```python
from build123d import *

# Parameters (mm, degrees)
SKETCH1_W                = 34
SKETCH1_H                = 28.5
BOSS_EXTRUDE1_DEPTH      = 22.7
SKETCH3_R                = 12.6
CUT_EXTRUDE1_DEPTH       = 21
SKETCH5_R                = 1.625
SKETCH5_R_2              = 3.75
CUT_EXTRUDE2_DEPTH       = 31.546071761
BOSS_EXTRUDE2_DEPTH      = 4.93
BOSS_EXTRUDE2_DEPTH_BACK = 3.72
SKETCH7_W                = 8.75
SKETCH7_H                = 12.5
SKETCH8_R                = 1.75
CUT_EXTRUDE3_DEPTH       = 42.018037496
SKETCH9_R                = 3.25
CUT_EXTRUDE4_DEPTH       = 3.175
SKETCH14_R               = 1.75
CUT_EXTRUDE8_DEPTH       = 50


with BuildPart() as part:
    # Sketch1 → Boss-Extrude1 (new body)
    with BuildSketch(Plane.XY):
        Rectangle(SKETCH1_W, SKETCH1_H)
    extrude(amount=BOSS_EXTRUDE1_DEPTH)

    # Sketch3 → Cut-Extrude1 (cut)
    with BuildSketch(Plane.XY.offset(22.7)):
        Circle(SKETCH3_R)
    extrude(amount=-CUT_EXTRUDE1_DEPTH, mode=Mode.SUBTRACT)

    # Sketch5 → Cut-Extrude2 (cut, through all)
    with BuildSketch(Plane.XY.offset(1.7)):
        with Locations((6.01040764, 6.01040764)):
            Circle(SKETCH5_R)
        with Locations((-6.01040764, 6.01040764)):
            Circle(SKETCH5_R)
        with Locations((6.01040764, -6.01040764)):
            Circle(SKETCH5_R)
        with Locations((-6.01040764, -6.01040764)):
            Circle(SKETCH5_R)
        Circle(SKETCH5_R_2)
    extrude(amount=-CUT_EXTRUDE2_DEPTH, mode=Mode.SUBTRACT)

    # Sketch7 → Boss-Extrude2 (add, two sides: drawn at the far end of the back side and taken through both)
    with BuildSketch(Plane.XY.offset(22.7).offset(-BOSS_EXTRUDE2_DEPTH_BACK)):
        with Locations((-21.375, -8)):
            Rectangle(SKETCH7_W, SKETCH7_H)
        with Locations((21.375, -8)):
            Rectangle(SKETCH7_W, SKETCH7_H)
    extrude(amount=BOSS_EXTRUDE2_DEPTH + BOSS_EXTRUDE2_DEPTH_BACK)

    # Sketch8 → Cut-Extrude3 (cut, through all)
    with BuildSketch(Plane(origin=(0, -1.75, 0), x_dir=(1, 0, 0), z_dir=(0, 1, 0))):
        with Locations(Location((21.375, -23.305, 0), (0, 0, 180))):
            Circle(SKETCH8_R)
        with Locations(Location((-21.375, -23.305, 0), (0, 0, 180))):
            Circle(SKETCH8_R)
    extrude(amount=-CUT_EXTRUDE3_DEPTH, mode=Mode.SUBTRACT)

    # Sketch9 → Cut-Extrude4 (cut)
    with BuildSketch(Plane.XZ.offset(14.25)):
        with Locations((-21.375, 23.305)):
            Circle(SKETCH9_R)
        with Locations((21.375, 23.305)):
            Circle(SKETCH9_R)
    extrude(amount=-CUT_EXTRUDE4_DEPTH, mode=Mode.SUBTRACT)

    # Cut-Extrude5 cone 1 section (through the dimple's axis) → Cut-Extrude5 (revolve, cut)
    with BuildSketch(Plane(origin=(-6.01040764, 6.01040764, 0), x_dir=(0, 1, 0), z_dir=(1, 0, 0))):
        Polygon((0, 0), (2.8, 0), (0, 2.8), align=None)
    revolve(axis=Axis((-6.01040764, 6.01040764, 0), (0, 0, 1)), mode=Mode.SUBTRACT)

    # Cut-Extrude5 cone 2 section (through the dimple's axis) → Cut-Extrude5 cone 2 (revolve, cut)
    with BuildSketch(Plane(origin=(-6.01040764, -6.01040764, 0), x_dir=(0, 1, 0), z_dir=(1, 0, 0))):
        Polygon((0, 0), (2.8, 0), (0, 2.8), align=None)
    revolve(axis=Axis((-6.01040764, -6.01040764, 0), (0, 0, 1)), mode=Mode.SUBTRACT)

    # Cut-Extrude5 cone 3 section (through the dimple's axis) → Cut-Extrude5 cone 3 (revolve, cut)
    with BuildSketch(Plane(origin=(6.01040764, -6.01040764, 0), x_dir=(0, 1, 0), z_dir=(1, 0, 0))):
        Polygon((0, 0), (2.8, 0), (0, 2.8), align=None)
    revolve(axis=Axis((6.01040764, -6.01040764, 0), (0, 0, 1)), mode=Mode.SUBTRACT)

    # Cut-Extrude5 cone 4 section (through the dimple's axis) → Cut-Extrude5 cone 4 (revolve, cut)
    with BuildSketch(Plane(origin=(6.01040764, 6.01040764, 0), x_dir=(0, 1, 0), z_dir=(1, 0, 0))):
        Polygon((0, 0), (2.8, 0), (0, 2.8), align=None)
    revolve(axis=Axis((6.01040764, 6.01040764, 0), (0, 0, 1)), mode=Mode.SUBTRACT)

    # Sketch14 → Cut-Extrude8 (cut)
    with BuildSketch(Plane(origin=(132.323959999, 1.25, 25.756345109), x_dir=(1, 0, 0), z_dir=(0, 1, 0))):
        with Locations((-110.733959999, 2.481345109)):
            Circle(SKETCH14_R)
        with Locations((-153.913959999, 2.481345109)):
            Circle(SKETCH14_R)
    extrude(amount=-CUT_EXTRUDE8_DEPTH, mode=Mode.SUBTRACT)


solid = part.part
```
Part model, mm, in its own coordinate system. A direction names the side the tool comes from. Round coordinates to 2 decimals unless told otherwise and drop trailing zeros. Write each loop counter-clockwise with the first axis right and the second up, starting at its lowest first coordinate (ties: lowest second). Pieces come first, ordered by that corner, then holes.
Item 1: Cut at C-C, the plane z = 26. Give the cut face in (x, y) (3 decimals), plus the area to 3 significant figures.
Results:
outline: (-25.75, -14.25) - (-23.191, -14.25) - (-23.191, -11.075) - (-19.559, -11.075) - (-19.559, -14.25) - (-17, -14.25) - (-17, -1.75) - (-25.75, -1.75) - close; (17, -14.25) - (19.559, -14.25) - (19.559, -11.075) - (23.191, -11.075) - (23.191, -14.25) - (25.75, -14.25) - (25.75, -1.75) - (17, -1.75) - close
area: 196 mm2
Item 2: Cut at A-A, the plane x = 0. Give the cut face in (y, z), plus the area to 3 significant figures.
Results:
outline: (-14.25, 0) - (-3.75, 0) - (-3.75, 1.7) - (-12.6, 1.7) - (-12.6, 22.7) - (-14.25, 22.7) - close; (3.75, 0) - (14.25, 0) - (14.25, 22.7) - (12.6, 22.7) - (12.6, 1.7) - (3.75, 1.7) - close
area: 105 mm2
Item 3: Cut at B-B, the plane y = 0. Give the cut face in (x, z), plus the area to 3 significant figures.
Results:
outline: (-17, 0) - (-3.75, 0) - (-3.75, 1.7) - (-12.6, 1.7) - (-12.6, 22.7) - (-17, 22.7) - close; (3.75, 0) - (17, 0) - (17, 22.7) - (12.6, 22.7) - (12.6, 1.7) - (3.75, 1.7) - close
area: 230 mm2
Item 4: Probe L1, parallel to Y at x = 0, z = 0.75; L2, parallel to X at y = -8.25, z = 26.5; L3, parallel to Z at x = 3.5, y = -1.75. List the from-to ranges inside material, lowest first.
Results:
L1: y = -14.25 to -3.75, 3.75 to 14.25
L2: x = -25.75 to -17, 17 to 25.75
L3: z = 0 to 1.7
Item 5: Which spindle directions (+Z, -Z, +X, -X, +Y, -Y) get a long thin tool onto all of the face, cutting with end or side? Do faces 4 (the cylindrical face through (20.67, -12.685, 20.132)), 5 (the flat face through (-21, -1.75, 21)), 6 (the flat face through (21, -8, 18.98)). Say none if no direction does.
Results:
face 4: -Y
face 5: +Z, -Z, -X, +Y
face 6: -Z, +X, +Y, -Y
Item 6: Drop flat-ended pins along their axis: pin 1 Ø4 at (x, y) = (16.5, 9.5) entering from +Z; pin 2 Ø5 at (x, y) = (-7, 5.5) entering from +Z; pin 3 Ø5 at (y, z) = (8, 6.5) entering from +X; pin 4 Ø2.5 at (x, y) = (-6.01, -6.01) entering from -Z. Give the stop position or say it passes through.
Results:
pin 1: stops at z = 22.7
pin 2: stops at z = 1.7
pin 3: stops at x = 17
pin 4: passes through
Item 7: Two-plate mould, pull along X, no slides. Class faces 1 (the flat face through (25.75, -8, 23)), 2 (the cylindrical face through (-9.999, -7.667, 12.347)), 3 (the flat face through (0, 14.25, 11)): +X half, -X half, draft (parallel to the pull), parting line (faces both ways), or undercut.
Results:
face 1: +X half
face 2: undercut
face 3: draft
Item 8: Cut at D-D, the plane z = 4. Give the cut face in (x, y), plus the area to 3 significant figures.
Results:
outline: (-17, -14.25) - (17, -14.25) - (17, 14.25) - (-17, 14.25) - close; hole circle Ø25.2 at (0, 0)
area: 470 mm2
